Design review of the part built by this model. Coordinates are the model's own, in mm. Face numbers are marked on the shaded views. Coordinates: 2 decimals unless noted, no trailing zeros. Write each loop counter-clockwise with the first axis right and the second up, starting at its lowest first coordinate (ties: lowest second). Pieces come first, ordered by that corner, then holes.
Q1. The part is to be moulded in two halves that separate along Z. For the marked faces 1, 2, 3 and 4, say which applies: +Z half, -Z half, draft (parallel to the pull), parting line (faces both ways), or undercut.
Q2. Clearance check with flat-ended pins moving along their axes: pin 1 Ø0.6 at (x, z) = (0.5, -1) entering from +Y; pin 2 Ø1 at (y, z) = (1, 1) entering from -X; pin 3 Ø0.5 at (y, z) = (-2.5, 0) entering from +X. State where each tip first meets the part, or that it passes through.
Q3. Add section C-C, the plane x = 0.55. Give the boundary of the cut face in (y, z), plus the area to 4 significant figures.
Q4. Add section D-D, the plane z = 0.5. Give the boundary of the cut face in (x, y).
Q5. Add section A-A, the plane y = -1. Give the number of separate pieces and of enclosed holes in the cut face, plus the area to 3 significant figures.
Q6. To check wall thickness, follow probe 1 along Y at (x, z) = (-0.9, -0.6); probe 2 along X at (y, z) = (1, 0.55). State the ranges of each line that lie inside material, in increasing order.
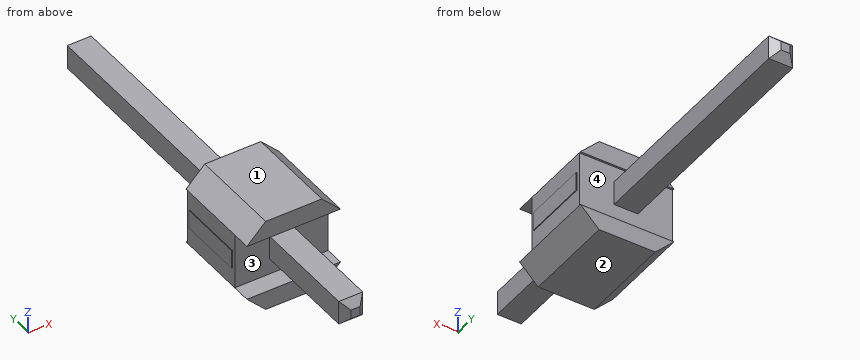
from build123d import *

# Parameters (mm, degrees)
SKETCH1_W           = 0.64
SKETCH1_H           = 11.54
BOSS_EXTRUDE1_DEPTH = 0.32
BOSS_EXTRUDE3_DEPTH = 1.25
CHAMFER1_SIZE       = 0.5
SKETCH3_W           = 0.5
SKETCH3_H           = 1.75
BOSS_EXTRUDE4_DEPTH = 1.27
CHAMFER2_SIZE       = 0.2


with BuildPart() as part:
    # Sketch1 → Boss-Extrude1 (new, symmetric)
    with BuildSketch(Plane(origin=(0, 0, 0), x_dir=(0, 0, -1), z_dir=(1, 0, 0))):
        with Locations((0, 1.98)):
            Rectangle(SKETCH1_W, SKETCH1_H)
    extrude(amount=BOSS_EXTRUDE1_DEPTH, both=True)

    # Sketch2 → Boss-Extrude3 (add, symmetric)
    with BuildSketch(Plane(origin=(0, 0, 0), x_dir=(0, -1, 0), z_dir=(1, 0, 0))):
        Polygon((-1.25, 1.25), (1.25, 1.25), (1.25, 0.75), (0.75, 0.75), (0.75, -0.75), (1.25, -0.75), (1.25, -1.25), (-1.25, -1.25), (-1.25, -0.75), (-1.2, -0.75), (-1.2, 0.75), (-1.25, 0.75), align=None)
    extrude(amount=BOSS_EXTRUDE3_DEPTH, both=True)

    # Chamfer1
    chamfer1_edges = [part.edges().sort_by_distance(p)[0] for p in [
        (1.25, 0, 1.25),
        (1.25, 0, -1.25),
        (-1.25, 0, 1.25),
        (-1.25, 0, -1.25),
    ]]
    chamfer(chamfer1_edges, length=CHAMFER1_SIZE - 0.0001)  # a hair under: the kernel refuses the full size

    # Sketch3 → Boss-Extrude4 (add, symmetric)
    with BuildSketch(Plane(origin=(0, 0, 0), x_dir=(0, 0, -1), z_dir=(1, 0, 0))):
        with Locations((0, 0.225)):
            Rectangle(SKETCH3_W, SKETCH3_H)
    extrude(amount=BOSS_EXTRUDE4_DEPTH, both=True)

    # Chamfer2
    chamfer2_edges = [part.edges().sort_by_distance(p)[0] for p in [
        (0.32, -3.79, 0),
        (0.32, 7.75, 0),
        (-0.32, -3.79, 0),
        (-0.32, 7.75, 0),
        (0, 7.75, -0.32),
        (0, -3.79, -0.32),
        (0, -3.79, 0.32),
        (0, 7.75, 0.32),
    ]]
    chamfer(chamfer2_edges, length=CHAMFER2_SIZE)


solid = part.part
Here are the results:
1. face 1: +Z half
1. face 2: -Z half
1. face 3: undercut
1. face 4: undercut
2. pin 1: stops at y = 1.25
2. pin 2: stops at x = -1.25
2. pin 3: stops at x = 0.32
3. outline: (-1.25, -1.25) - (1.25, -1.25) - (1.25, -0.75) - (1.2, -0.75) - (1.2, 0.75) - (1.25, 0.75) - (1.25, 1.25) - (-1.25, 1.25) - (-1.25, 0.75) - (-0.75, 0.75) - (-0.75, -0.75) - (-1.25, -0.75) - close
3. area: 5.425 mm2
4. outline: (-1.25, -0.75) - (1.25, -0.75) - (1.25, 1.2) - (-1.25, 1.2) - close
5. separate pieces: 3
5. enclosed holes: 0
5. area: 2.41 mm2
6. probe 1: y = -0.75 to 1.2
6. probe 2: x = -1.25 to 1.25
